Read the model definition and answer for the solid it produces. Units are mm, in the model's axes. Coordinates: 2 decimals unless noted, no trailing zeros. Order: outer loops, then holes, each group sorted by start corner. A loop starts at its lowest first (then second) coordinate and runs counter-clockwise, first axis right, second up. Notation, with made-up numbers: (83, 85) -> (137, 85) arc R26 cw to (137, 114) -> close; hole circle Ø1 at (19.5, 24.5). An arc over 180 degrees is marked (long way). Answer in a Markdown table with one row per item.
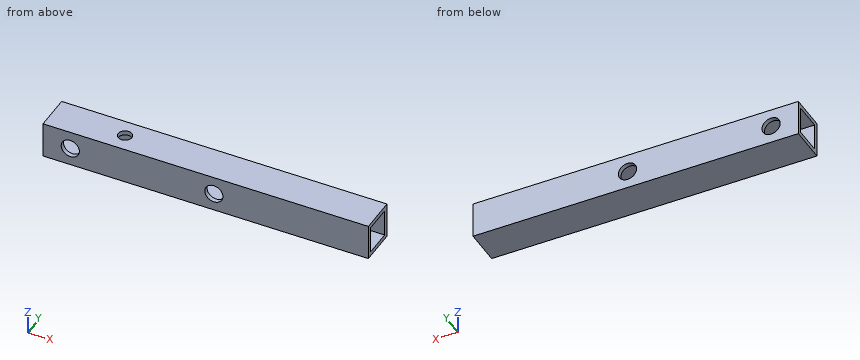
Autodesk Inventor part; units mm, degrees
ref_plane "YZ Plane" through (0, 0, 0) normal (1, 0, 0) x (0, 1, 0)
ref_plane "XZ Plane" through (0, 0, 0) normal (0, 1, 0) x (-1, 0, 0)
ref_plane "XY Plane" through (0, 0, 0) normal (0, 0, 1) x (1, 0, 0)
sketch "Sketch1" plane through (0, 0, 0) normal (1, 0, 0) x (0, 1, 0)
  line L0 (0, 0) -> (25.4, 0)
  line L1 (25.4, 0) -> (25.4, 25.4)
  line L2 (25.4, 25.4) -> (0, 25.4)
  line L3 (0, 25.4) -> (0, 0)
  line L4 (3.175, 22.225) -> (22.225, 22.225)
  line L5 (22.225, 22.225) -> (22.225, 3.175)
  line L6 (22.225, 3.175) -> (3.175, 3.175)
  line L7 (3.175, 3.175) -> (3.175, 22.225)
  dimension "d0" = 25.4
  dimension "d1" = 25.4
  dimension "d2" = 3.175
extrude "Extrusion1" add sketch "Sketch1" along normal blind 227.33
sketch "Sketch2" plane through (0, 25.4, 25.4) normal (0, 1, 0) x (1, 0, 0)
  line L0 (0, 25.4) -> (0, 0)
  line L1 (0, 25.4) -> (227.33, 25.4)
  circle A0 centre (19.05, 12.7) radius 6.35
  dimension "d5" = 12.7
  dimension "d6" = 12.7
  dimension "d7" = 19.05
extrude "Extrusion2" cut sketch "Sketch2" against normal blind 25.4
sketch "Sketch3" plane through (0, 0, 25.4) normal (0, 0, 1) x (1, 0, 0)
  line L0 (0, 25.4) -> (0, 0)
  line L1 (0, 25.4) -> (227.33, 25.4)
  circle A0 centre (50.8, 12.7) radius 4.7625
  dimension "d10" = 9.525
  dimension "d11" = 50.8
  dimension "d12" = 12.7
extrude "Extrusion3" cut sketch "Sketch3" against normal up to next
sketch "Sketch4" plane through (0, 25.4, 25.4) normal (0, 1, 0) x (1, 0, 0)
  line L0 (227.33, 25.4) -> (227.33, 0)
  line L1 (0, 25.4) -> (227.33, 25.4)
  point P0 (119.38, 12.7)
  dimension "d15" = 12.7
  dimension "d16" = 107.95
hole "Hole1" at (119.38, 25.4, 12.7) direction (0, -1, 0) diameter 12.7 end through all
properties part number "Box 9 inch" material "Aluminum 6061"
Q1. The part is cut by section B-B (x = 174). Write down the section's boundary in (y, z) (3 decimals).
Outcome:
| item | result |
|---|---|
| outline | (0, 0) -> (25.4, 0) -> (25.4, 25.4) -> (0, 25.4) -> close; hole (3.175, 3.175) -> (22.225, 3.175) -> (22.225, 22.225) -> (3.175, 22.225) -> close |
Q2. Given pin 1 (7.5 mm diameter, centred on x = 19.05, z = 12.7, fed in from -Y), flat-ended and moving along its own axis, determine where the tip first touches the part or whether it passes through.
Outcome:
| item | result |
|---|---|
| pin 1 | through |
Q3. The part is cut by section D-D (x = 50.8). Write down the section's boundary in (y, z) (1 decimal).
Outcome:
| item | result |
|---|---|
| outline | (0, 0) -> (25.4, 0) -> (25.4, 25.4) -> (17.5, 25.4) -> (17.5, 22.2) -> (22.2, 22.2) -> (22.2, 3.2) -> (3.2, 3.2) -> (3.2, 22.2) -> (7.9, 22.2) -> (7.9, 25.4) -> (0, 25.4) -> close |
Q4. The part is cut by section A-A (y = 12.7). Write down the section's boundary in (x, z) (1 decimal).
Outcome:
| item | result |
|---|---|
| outline | (0, 0) -> (227.3, 0) -> (227.3, 3.2) -> (0, 3.2) -> close; (0, 22.2) -> (46, 22.2) -> (46, 25.4) -> (0, 25.4) -> close; (55.6, 22.2) -> (227.3, 22.2) -> (227.3, 25.4) -> (55.6, 25.4) -> close |
Q5. The part is cut by section C-C (x = 19.05). Write down the section's boundary in (y, z) (3 decimals), then the cut area to 3 significant figures.
Outcome:
| item | result |
|---|---|
| outline | (0, 0) -> (25.4, 0) -> (25.4, 6.35) -> (22.225, 6.35) -> (22.225, 3.175) -> (3.175, 3.175) -> (3.175, 6.35) -> (0, 6.35) -> close; (0, 19.05) -> (3.175, 19.05) -> (3.175, 22.225) -> (22.225, 22.225) -> (22.225, 19.05) -> (25.4, 19.05) -> (25.4, 25.4) -> (0, 25.4) -> close |
| area | 202 mm² |
Q6. Consider line 1 (X direction, y = 1.5, z = 13.25); line 2 (Z direction, x = 76, y = 9.75) (3 decimals). Determine where each line is inside the solid, lowest interval first.
Outcome:
| item | result |
|---|---|
| line 1 | 0 to 12.72, 25.38 to 113.05, 125.71 to 227.33 |
| line 2 | 0 to 3.175, 22.225 to 25.4 |
